from build123d import *

# Parameters (mm, degrees)
F0_W     = 25.4
F0_H     = 50.8
F1_DEPTH = 50.8
F2_R     = 12.7
F3_DEPTH = 25.401
F5_D     = 5.1054
F5_DEPTH = 12.7
F5_TIP   = 1.5338169022


with BuildPart() as f1:
    # F0 (on Front) → F1 (new body)
    with BuildSketch(Plane.XZ):
        with Locations((12.7, 25.4)):
            Rectangle(F0_W, F0_H)
    extrude(amount=F1_DEPTH)

    # F2 (on face) → F3 (cut, through all)
    with BuildSketch(Plane.YZ.offset(25.4)):
        with Locations((-25.4, 25.4)):
            Circle(F2_R)
    extrude(amount=-F3_DEPTH, mode=Mode.SUBTRACT)

    # F5
    with Locations(Plane.XY.offset(50.8)):
        with Locations((12.7, -25.4)):
            Hole(F5_D / 2, depth=F5_DEPTH)
            with Locations((0, 0, -(F5_DEPTH + F5_TIP / 2))):  # 118° drill point
                Cone(0, F5_D / 2, F5_TIP, mode=Mode.SUBTRACT)


solid = f1.part
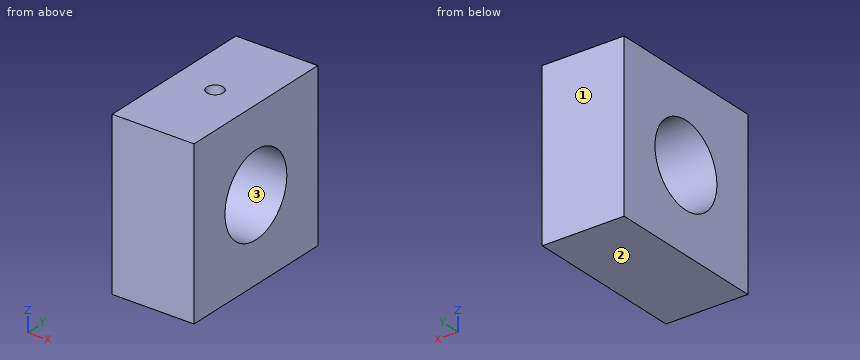
The listing builds one solid part. Answer for the finished solid, in the listing's coordinates (mm). Face numbers are marked on the shaded views. Coordinates: 2 decimals unless noted, no trailing zeros. Order: outer loops, then holes, each group sorted by start corner. A loop starts at its lowest first (then second) coordinate and runs counter-clockwise, first axis right, second up.
Q1. Consider line 1 (Y direction, x = 12.75, z = 41); line 2 (Z direction, x = 20, y = -14); line 3 (Z direction, x = 8, y = -18.5). Determine where each line is inside the solid, lowest interval first.
Q2. A cutting plane is placed at C-C, the plane y = -33.5. Write down the section's boundary in (x, z), and give its area (3 significant figures).
Q3. A cutting plane is placed at A-A, the plane z = 25.4. Write down the section's boundary in (x, y).
Q4. A cutting plane is placed at D-D, the plane z = 40. Write down the section's boundary in (x, y).
Q5. A cutting plane is placed at B-B, the plane x = 23.75. Write down the section's boundary in (y, z).
Q6. For a pull along Y with two mould halves and no side action, classify the marked faces 1, 2 and 3 as pulls with the +Y half, pulls with the -Y half, needs draft (parallel to the pull), parting line crosses it, or undercut.
Answers follow:
1. line 1: y = -50.8 to -27.95, -22.85 to 0
1. line 2: z = 0 to 19.8, 31 to 50.8
1. line 3: z = 0 to 14.74, 36.06 to 50.8
2. outline: (0, 0) - (25.4, 0) - (25.4, 15.62) - (0, 15.62) - close; (0, 35.18) - (25.4, 35.18) - (25.4, 50.8) - (0, 50.8) - close
2. area: 793 mm2
3. outline: (0, -50.8) - (25.4, -50.8) - (25.4, -38.1) - (0, -38.1) - close; (0, -12.7) - (25.4, -12.7) - (25.4, 0) - (0, 0) - close
4. outline: (0, -50.8) - (25.4, -50.8) - (25.4, 0) - (0, 0) - close; hole circle Ø5.11 at (12.7, -25.4)
5. outline: (-50.8, 0) - (0, 0) - (0, 50.8) - (-50.8, 50.8) - close; hole circle Ø25.4 at (-25.4, 25.4)
6. face 1: pulls with the +Y half
6. face 2: needs draft
6. face 3: undercut
